Source: CAD feature listing. Evaluate the final solid. Frame: model axes, mm. Give positions to 0.01 mm unless a question says otherwise; leave off trailing zeros. Loops run counter-clockwise (first coordinate to the right, second up) from the corner with the lowest first, then second, coordinate; pieces in that order, holes last. Notation, with made-up numbers: (-9.5, -32) -> (45.5, -32) arc R32 ccw to (45.5, -4) -> close; hole circle Ø2 at (77.5, 16). An arc over 180 degrees is marked (long way). Put each result on its own line as item: value.
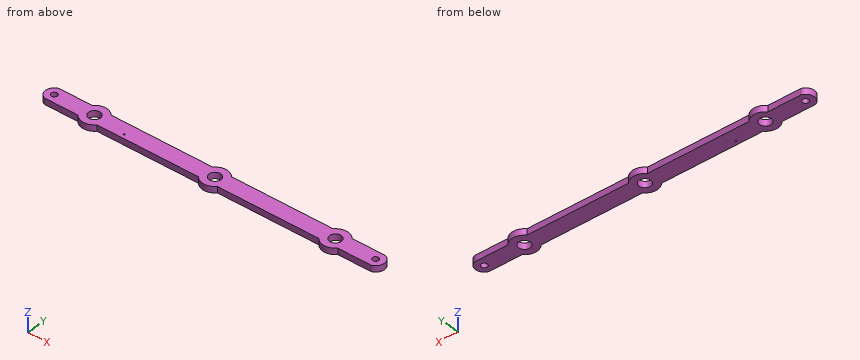
```python
from build123d import *

# Parameters (mm, degrees)
SKETCH1_R           = 2.9
SKETCH1_R_2         = 1.5
SKETCH1_R_3         = 0.390297289
BOSS_EXTRUDE1_DEPTH = 3


with BuildPart() as part:
    # Sketch1 → Boss-Extrude1 (new body)
    with BuildSketch(Plane.XY):
        with BuildLine():
            Line((-81.201730293, 4.097407022), (-64.706257079, 4.097407022))
            ThreePointArc((-64.706257079, 4.097407022), (-60, 6.24), (-55.293742921, 4.097407022))
            Line((-55.293742921, 4.097407022), (-4.706257079, 4.097407022))
            ThreePointArc((-4.706257079, 4.097407022), (0, 6.24), (4.706257079, 4.097407022))
            Line((4.706257079, 4.097407022), (55.293742921, 4.097407022))
            ThreePointArc((55.293742921, 4.097407022), (60, 6.24), (64.706257079, 4.097407022))
            Line((64.706257079, 4.097407022), (81.201730293, 4.097407022))
            ThreePointArc((81.201730293, 4.097407022), (84.27, 0), (81.201730293, -4.097407022))
            Line((81.201730293, -4.097407022), (64.706257079, -4.097407022))
            ThreePointArc((64.706257079, -4.097407022), (60, -6.24), (55.293742921, -4.097407022))
            Line((55.293742921, -4.097407022), (4.706257079, -4.097407022))
            ThreePointArc((4.706257079, -4.097407022), (0, -6.24), (-4.706257079, -4.097407022))
            Line((-4.706257079, -4.097407022), (-55.293742921, -4.097407022))
            ThreePointArc((-55.293742921, -4.097407022), (-60, -6.24), (-64.706257079, -4.097407022))
            Line((-64.706257079, -4.097407022), (-81.201730293, -4.097407022))
            ThreePointArc((-81.201730293, -4.097407022), (-84.27, 0), (-81.201730293, 4.097407022))
        make_face()
        with Locations((-60, 0)):
            Circle(SKETCH1_R, mode=Mode.SUBTRACT)
        Circle(SKETCH1_R, mode=Mode.SUBTRACT)
        with Locations((60, 0)):
            Circle(SKETCH1_R, mode=Mode.SUBTRACT)
        with Locations((80, 0)):
            Circle(SKETCH1_R_2, mode=Mode.SUBTRACT)
        with Locations((-80, 0)):
            Circle(SKETCH1_R_2, mode=Mode.SUBTRACT)
        with Locations((-43.533553558, -1.94889321)):
            Circle(SKETCH1_R_3, mode=Mode.SUBTRACT)
    extrude(amount=BOSS_EXTRUDE1_DEPTH)


solid = part.part
```
(1) Section D-D on x = 45.5. Return loops of the section in (y, z), then the cut area to 3 significant figures.
Calculated:
outline: (-4.1, 0) -> (4.1, 0) -> (4.1, 3) -> (-4.1, 3) -> close
area: 24.6 mm²
(2) First-contact query: P1, Ø0.9, axis at x = -33.5, z = 1, coming from the +Y side; P2, Ø4.5, axis at x = 60, y = 0, coming from the -Z side. Flat tips, straight axial feed; report the tip coordinate or a pass-through.
Calculated:
P1: stops at y = 4.1
P2: passes through
(3) Line query: probe 1 along Y at (x, z) = (-60, 0.9); probe 2 along X at (y, z) = (-2.25, 0.25); probe 3 along X at (y, z) = (-2.5, 0.65). Output: solid intervals per line, ascending. Write a range as from..to.
Calculated:
probe 1: y = -6.24..-2.9, 2.9..6.24
probe 2: x = -83.63..-61.83, -58.17..-43.78, -43.29..-1.83, 1.83..58.17, 61.83..83.63
probe 3: x = -83.46..-61.47, -58.53..-1.47, 1.47..58.53, 61.47..83.46
(4) Section C-C on z = 1.65. Return loops of the section in (x, y).
Calculated:
outline: (-81.2, -4.1) -> (-64.71, -4.1) arc R6.24 ccw to (-55.29, -4.1) -> (-4.71, -4.1) arc R6.24 ccw to (4.71, -4.1) -> (55.29, -4.1) arc R6.24 ccw to (64.71, -4.1) -> (81.2, -4.1) arc R4.27 ccw to (81.2, 4.1) -> (64.71, 4.1) arc R6.24 ccw to (55.29, 4.1) -> (4.71, 4.1) arc R6.24 ccw to (-4.71, 4.1) -> (-55.29, 4.1) arc R6.24 ccw to (-64.71, 4.1) -> (-81.2, 4.1) arc R4.27 ccw to start; hole circle Ø3 at (-80, 0); hole circle Ø5.8 at (-60, 0); hole circle Ø0.78 at (-43.53, -1.95); hole circle Ø5.8 at (0, 0); hole circle Ø5.8 at (60, 0); hole circle Ø3 at (80, 0)
(5) Section B-B on y = 0. Return loops of the section in (x, z), then the cut area to 3 significant figures.
Calculated:
outline: (-84.27, 0) -> (-81.5, 0) -> (-81.5, 3) -> (-84.27, 3) -> close; (-78.5, 0) -> (-62.9, 0) -> (-62.9, 3) -> (-78.5, 3) -> close; (-57.1, 0) -> (-2.9, 0) -> (-2.9, 3) -> (-57.1, 3) -> close; (2.9, 0) -> (57.1, 0) -> (57.1, 3) -> (2.9, 3) -> close; (62.9, 0) -> (78.5, 0) -> (78.5, 3) -> (62.9, 3) -> close; (81.5, 0) -> (84.27, 0) -> (84.27, 3) -> (81.5, 3) -> close
area: 435 mm²
(6) Section A-A on x = -60. Return loops of the section in (y, z), then the cut area to 3 significant figures.
Calculated:
outline: (-6.24, 0) -> (-2.9, 0) -> (-2.9, 3) -> (-6.24, 3) -> close; (2.9, 0) -> (6.24, 0) -> (6.24, 3) -> (2.9, 3) -> close
area: 20.0 mm²
